Work out the finished part from the listing and answer in its coordinate system (mm). Coordinates: 2 decimals unless noted, no trailing zeros. Order: outer loops, then holes, each group sorted by start corner. A loop starts at its lowest first (then second) coordinate and runs counter-clockwise, first axis right, second up. Notation, with made-up numbers: (51.25, 10) -> (85.25, 10) arc R29 ccw to (85.25, 31) -> close; hole circle Ø11 at (-39, 33). An arc over 180 degrees is marked (long way). Answer as CSV lines item,"result". Start each with the question number.
Item 1: For a pull along Y with two mould halves and no side action, classify faces 1 (the face through (99, 106, 0)), 2 (the face through (102, 208.28, 6)), 3 (the face through (179.86, 31.93, 6.44)), 4 (the face through (20.61, 33, 6.44)) as pulls with the +Y half, pulls with the -Y half, needs draft (parallel to the pull), parting line crosses it, or undercut.
Item 2: This flat-tipped pin is pushed along its axis until it touches: pin 1 Ø1.5 at (x, z) = (166, 6.5) entering from -Y. Where does it stop, or does it pass through?
Item 3: Section A-A (y = 31.75) is taken. Write down the section's boundary in (x, z).
Autodesk Inventor part; units mm, degrees
ref_plane "YZ Plane" through (0, 0, 0) normal (1, 0, 0) x (0, 1, 0)
ref_plane "XZ Plane" through (0, 0, 0) normal (0, 1, 0) x (-1, 0, 0)
ref_plane "XY Plane" through (0, 0, 0) normal (0, 0, 1) x (1, 0, 0)
sketch "Sketch1" plane through (0, 0, 0) normal (0, 0, 1) x (1, 0, 0)
  line L0 (0, 0) -> (200.66, 0)
  line L1 (200.66, 0) -> (200.66, 208.28)
  line L2 (200.66, 208.28) -> (0, 208.28)
  line L3 (0, 208.28) -> (0, 0)
  dimension "d0" = 200.66
  dimension "d1" = 208.28
extrude "Extrusion1" add sketch "Sketch1" along normal blind 12.7
sketch "Sketch2" plane through (0, 0, 12.7) normal (0, 0, 1) x (1, 0, 0)
  circle A0 centre (184.023, 31.75) radius 4.1656
  line L0 (0, 0) -> (200.66, 0)
  line L1 (200.66, 0) -> (200.66, 208.28)
  circle A1 centre (16.637, 31.75) radius 4.1656
  line L2 (0, 208.28) -> (0, 0)
  dimension "d4" = 8.3312
  dimension "d5" = 31.75
  dimension "d6" = 16.637
  dimension "d7" = 8.3312
  dimension "d8" = 16.637
  dimension "d9" = 31.75
extrude "Extrusion2" cut sketch "Sketch2" against normal blind 25.4
properties part number "Side wall"
Checked values:
1,face 1,"needs draft"
1,face 2,"pulls with the +Y half"
1,face 3,"undercut"
1,face 4,"undercut"
2,pin 1,"stops at y = 0"
3,outline,"(0, 0) -> (12.47, 0) -> (12.47, 12.7) -> (0, 12.7) -> close; (20.8, 0) -> (179.86, 0) -> (179.86, 12.7) -> (20.8, 12.7) -> close; (188.19, 0) -> (200.66, 0) -> (200.66, 12.7) -> (188.19, 12.7) -> close"
